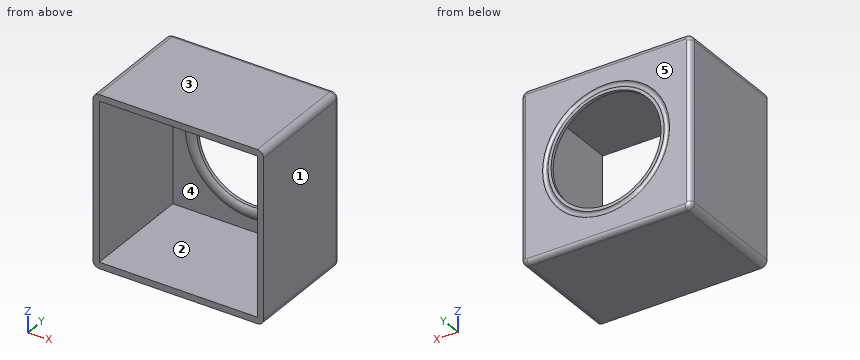
from build123d import *

# Parameters (mm, degrees)
SKETCH1_W               = 99.503865414
SKETCH1_H               = 99.503865414
BOSS_EXTRUDE1_DEPTH     = 70
BOSS_EXTRUDE2_OUTLINE_R = 41.055084084
BOSS_EXTRUDE2_DEPTH     = 2
FILLET1_R               = 3


# Read off the part's stored shape, not the designer's step: Boss-Extrude2
with BuildPart() as part:
    # Sketch1 → Boss-Extrude1 (new body)
    with BuildSketch(Plane(origin=(0, 0, 0), x_dir=(1, 0, 0), z_dir=(0, 1, 0))):
        with BuildLine():
            Line((-49.751932707, -53.751932707), (49.751932707, -53.751932707))
            ThreePointArc((49.751932707, -53.751932707), (52.580359832, -52.580359832), (53.751932707, -49.751932707))
            Line((53.751932707, -49.751932707), (53.751932707, 49.751932707))
            ThreePointArc((53.751932707, 49.751932707), (52.580359832, 52.580359832), (49.751932707, 53.751932707))
            Line((49.751932707, 53.751932707), (-49.751932707, 53.751932707))
            ThreePointArc((-49.751932707, 53.751932707), (-52.580359832, 52.580359832), (-53.751932707, 49.751932707))
            Line((-53.751932707, 49.751932707), (-53.751932707, -49.751932707))
            ThreePointArc((-53.751932707, -49.751932707), (-52.580359832, -52.580359832), (-49.751932707, -53.751932707))
        make_face()
        Rectangle(SKETCH1_W, SKETCH1_H, mode=Mode.SUBTRACT)
    extrude(amount=BOSS_EXTRUDE1_DEPTH)

    # Boss-Extrude2 outline → Boss-Extrude2 (add)
    with BuildSketch(Plane(origin=(0, 70, 0), x_dir=(1, 0, 0), z_dir=(0, 1, 0))):
        with BuildLine():
            ThreePointArc((-53.751932707, -49.751932707), (-52.580359832, -52.580359832), (-49.751932707, -53.751932707))
            Line((-49.751932707, -53.751932707), (49.751932707, -53.751932707))
            ThreePointArc((49.751932707, -53.751932707), (52.580359832, -52.580359832), (53.751932707, -49.751932707))
            Line((53.751932707, -49.751932707), (53.751932707, 49.751932707))
            ThreePointArc((53.751932707, 49.751932707), (52.580359832, 52.580359832), (49.751932707, 53.751932707))
            Line((49.751932707, 53.751932707), (-49.751932707, 53.751932707))
            ThreePointArc((-49.751932707, 53.751932707), (-52.580359832, 52.580359832), (-53.751932707, 49.751932707))
            Line((-53.751932707, 49.751932707), (-53.751932707, -49.751932707))
        make_face()
        Circle(BOSS_EXTRUDE2_OUTLINE_R, mode=Mode.SUBTRACT)
    extrude(amount=BOSS_EXTRUDE2_DEPTH)

    # Fillet1
    fillet1_edges = [part.edges().sort_by_distance(p)[0] for p in [
        (-53.751932707, 72, 0),
        (-52.580359832, 72, 52.580359832),
        (0, 72, 53.751932707),
        (52.580359832, 72, 52.580359832),
        (53.751932707, 72, 0),
        (52.580359832, 72, -52.580359832),
        (0, 72, -53.751932707),
        (-52.580359832, 72, -52.580359832),
    ]]
    fillet(fillet1_edges, radius=FILLET1_R)

    # Sketch6 → Revolve1 (revolve)
    with BuildSketch(Plane(origin=(0, 0, 0), x_dir=(0, 0, -1), z_dir=(1, 0, 0)), mode=Mode.PRIVATE) as revolve1_sk:
        with BuildLine():
            Line((-41.906282127, 70), (-41.906282127, 72))
            Line((-41.906282127, 72), (-39.977926792, 72))
            ThreePointArc((-39.977926792, 72), (-38.268844469, 71.01399696), (-36.559762147, 72))
            Line((-36.559762147, 72), (-34.631406812, 72))
            Line((-34.631406812, 72), (-34.631406812, 70))
            ThreePointArc((-34.631406812, 70), (-38.268844469, 68.645456934), (-41.906282127, 70))
        make_face()
    revolve(revolve1_sk.sketch.rotate(Axis((0, 0, 0), (0, 1, 0)), 180), axis=Axis((0, 0, 0), (0, 1, 0)))


solid = part.part
Model file for the job. Use its own axes, mm. Face numbers are marked on the shaded views. A direction names the side the tool comes from. Give positions to 0.01 mm unless a question says otherwise; leave off trailing zeros. Order: outer loops, then holes, each group sorted by start corner. A loop starts at its lowest first (then second) coordinate and runs counter-clockwise, first axis right, second up. Notation, with made-up numbers: (32.5, 40.5) - (36.5, 40.5) arc R15 cw to (36.5, 62.5) - close; hole circle Ø7 at (-7.5, 43). An arc over 180 degrees is marked (long way). Return JSON: item names as keys, results as strings.
1) Pull direction Z, two halves, no side cores. Call the marked faces 1, 2 and 3: pulls with the +Z half, pulls with the -Z half, needs draft (parallel to the pull), parting line crosses it, or undercut.
Geometry says:
{"face 1": "needs draft", "face 2": "undercut", "face 3": "pulls with the +Z half"}
2) Cut at C-C, the plane y = 12. Give the cut face in (x, z), plus the area to 3 significant figures.
Geometry says:
{"outline": "(-53.75, -49.75) arc R4 ccw to (-49.75, -53.75) - (49.75, -53.75) arc R4 ccw to (53.75, -49.75) - (53.75, 49.75) arc R4 ccw to (49.75, 53.75) - (-49.75, 53.75) arc R4 ccw to (-53.75, 49.75) - close; hole (-49.75, -49.75) - (49.75, -49.75) - (49.75, 49.75) - (-49.75, 49.75) - close", "area": "1,640 mm²"}
3) Cut at A-A, the plane x = 0. Give the cut face in (y, z), plus the area to 3 significant figures.
Geometry says:
{"outline": "(0, -53.75) - (69, -53.75) arc R3 ccw to (72, -50.75) - (72, -39.98) arc R1.97 cw to (72, -36.56) - (72, -34.63) - (70, -34.63) arc R5.56 ccw to (70, -41.91) - (70, -49.75) - (0, -49.75) - close; (0, 49.75) - (70, 49.75) - (70, 41.91) arc R5.56 ccw to (70, 34.63) - (72, 34.63) - (72, 36.56) arc R1.97 cw to (72, 39.98) - (72, 50.75) arc R3 ccw to (69, 53.75) - (0, 53.75) - close", "area": "641 mm²"}
4) Cut at B-B, the plane z = 0. Give the cut face in (x, y), plus the area to 3 significant figures.
Geometry says:
{"outline": "(-53.75, 0) - (-49.75, 0) - (-49.75, 70) - (-41.91, 70) arc R5.56 ccw to (-34.63, 70) - (-34.63, 72) - (-36.56, 72) arc R1.97 cw to (-39.98, 72) - (-50.75, 72) arc R3 ccw to (-53.75, 69) - close; (34.63, 70) arc R5.56 ccw to (41.91, 70) - (49.75, 70) - (49.75, 0) - (53.75, 0) - (53.75, 69) arc R3 ccw to (50.75, 72) - (39.98, 72) arc R1.97 cw to (36.56, 72) - (34.63, 72) - close", "area": "641 mm²"}
5) Probe line 1 (Z direction, x = -3, y = 22); line 2 (Z direction, x = 4, y = 69.5). List the from-to ranges inside material, lowest first. Write a range as from..to.
Geometry says:
{"line 1": "-53.75..-49.75, 49.75..53.75", "line 2": "-53.71..-49.75, -41.04..-35.08, 35.08..41.04, 49.75..53.71"}
6) 3-axis set-ups, long thin cutter, end or side, ignore diameter. For the marked faces 4 and 5: which of +Z, -Z, +X, -X, +Y, -Y reach the whole face in a straight line?
Geometry says:
{"face 4": "-Y", "face 5": "+Z, -Z, +X, -X, +Y"}
